```python
from build123d import *

# Parameters (mm, degrees)
F0_R     = 40.000185
F1_DEPTH = 10
F2_R     = 2.50061
F3_DEPTH = 50
F4_R     = 2.501284
F4_R_2   = 2.498539
F4_R_3   = 2.501993
F4_R_4   = 2.501243
F5_DEPTH = 50


with BuildPart() as f1:
    # F0 (on Top) → F1 (new body)
    with BuildSketch(Plane.XY):
        Circle(F0_R)
    extrude(amount=F1_DEPTH)

    # F2 (on face) → F3 (join)
    with BuildSketch(Plane.XY.offset(10)):
        Circle(F2_R)
    extrude(amount=F3_DEPTH)

    # F4 (on face) → F5 (join)
    with BuildSketch(Plane.XY.offset(10)):
        with Locations((0, 35.487343)):
            Circle(F4_R)
        with Locations((-35.967495, 0)):
            Circle(F4_R_2)
        with Locations((0, -35.491817)):
            Circle(F4_R_3)
        with Locations((35.982933, 0)):
            Circle(F4_R_4)
    extrude(amount=F5_DEPTH)


solid = f1.part
```
Design review of the part built by this model. Coordinates are the model's own, in mm. A direction names the side the tool comes from. Coordinates: 2 decimals unless noted, no trailing zeros. Order: outer loops, then holes, each group sorted by start corner. A loop starts at its lowest first (then second) coordinate and runs counter-clockwise, first axis right, second up. Notation, with made-up numbers: M 10.5,21 L 22.5,21 A18 cw 22.5,55 Z; hole C 56.25,22.5 d6. An arc over 180 degrees is marked long. Answer as a JSON object with one key per item and string values. Group by question number.
1) Tool access review of faces 1 (the flat face through (-1, -8, 10)), 2 (the flat face through (0, 36, 60)): name each direction out of +Z, -Z, +X, -X, +Y, -Y from which nothing blocks a thin tool from reaching the whole face with its end or side.
2) Add section D-D, the plane y = 29. Write out the cut boundary in (x, z).
3) For pin 1 (2 mm diameter, centred on y = 14, z = 9.5, fed in from -X); pin 2 (10 mm diameter, centred on x = 6.5, y = 18, fed in from -Z); pin 3 (12 mm diameter, centred on x = 1, y = 9.5, fed in from +Z); pin 4 (4 mm diameter, centred on y = -3, z = 47.5, fed in from -X), all flat-tipped, find the tip position at first contact; note any pin that passes through.
4) Mouldability with a two-part tool opening along Y and no side actions: class faces 3 (the cylindrical face through (1.154, 33.268, 34.65)), 4 (the cylindrical face through (-33.66, -0.96, 34.65)), 5 (the flat face through (0, -35, 60)) as pulls with the +Y half, pulls with the -Y half, needs draft (parallel to the pull), parting line crosses it, or undercut.
5) Add section C-C, the plane z = 56. Write out the cut boundary in (x, y), then the cut area to 3 significant figures.
6) Add section A-A, the plane x = 0. Write out the cut boundary in (y, z).
7) Add section B-B, the plane y = 0. Write out the cut boundary in (x, z).
8) Wall thickness on L1, parallel to Y at x = 0, z = 49.5; L2, parallel to Z at x = 25, y = -27.5; L3, parallel to X at y = -0.5, z = 21: over which ranges is each line inside the solid? List them lowest first.
Computed values:
{
 "1": {"face 1": "+Z", "face 2": "+Z, +X, -X, +Y, -Y"},
 "2": {"outline": "M -27.55,0 L 27.55,0 L 27.55,10 L -27.55,10 Z"},
 "3": {"pin 1": "stops at x = -37.83", "pin 2": "stops at z = 0", "pin 3": "stops at z = 10", "pin 4": "stops at x = -38.26"},
 "4": {"face 3": "undercut", "face 4": "parting line crosses it", "face 5": "needs draft"},
 "5": {"outline": "C -35.97,0 d5; C 0,-35.49 d5; C 0,0 d5; C 0,35.49 d5; C 35.98,0 d5", "area": "98.2 mm^2"},
 "6": {"outline": "M -40,0 L 40,0 L 40,10 L 37.99,10 L 37.99,60 L 32.99,60 L 32.99,10 L 2.5,10 L 2.5,60 L -2.5,60 L -2.5,10 L -32.99,10 L -32.99,60 L -37.99,60 L -37.99,10 L -40,10 Z"},
 "7": {"outline": "M -40,0 L 40,0 L 40,10 L 38.48,10 L 38.48,60 L 33.48,60 L 33.48,10 L 2.5,10 L 2.5,60 L -2.5,60 L -2.5,10 L -33.47,10 L -33.47,60 L -38.47,60 L -38.47,10 L -40,10 Z"},
 "8": {"L1": "y = -37.99 to -32.99, -2.5 to 2.5, 32.99 to 37.99", "L2": "z = 0 to 10", "L3": "x = -38.42 to -33.52, -2.45 to 2.45, 33.53 to 38.43"}
}
